The drawing under review shows one solid part. Ordinate dimensions are in mm from its lowest x, y, z. A direction names the side the tool comes from. Give positions to 0.01 mm unless a question says otherwise; leave off trailing zeros. Loops run counter-clockwise (first coordinate to the right, second up) from the corner with the lowest first, then second, coordinate; pieces in that order, holes last. Notation, with made-up numbers: M -29,81 L -11,81 A37 cw -11,117 Z; hole C -17,-24 d11. An arc over 180 degrees is marked long. One line per item, written item: value. Start each with the question number.
Q1. We need section C-C on x = 5. Write out the cut boundary in (y, z), plus the area to 3 significant figures.
Q2. We need section D-D on y = 4.5. Write out the cut boundary in (x, z), plus the area to 3 significant figures.
Q3. We need section A-A on z = 15. Write out the cut boundary in (x, y).
Q4. For pin 1 (1 mm diameter, centred on x = 15, z = 5, fed in from -Y); pin 2 (2.5 mm diameter, centred on x = 5, z = 15, fed in from +Y); pin 3 (3 mm diameter, centred on y = 15.5, z = 3.5, fed in from -X); pin 4 (2 mm diameter, centred on y = 5, z = 10.5, fed in from -X), all flat-tipped, find the tip position at first contact; note any pin that passes through.
Q5. To check wall thickness, follow line 1 along Z through (x, y) = (15, 16.75); line 2 along Z through (x, y) = (15.5, 12.5); line 3 along Y through (x, z) = (10.5, 18.25). State the ranges of each line that lie inside material, in increasing order. Write a range as from..to.
Q6. Mouldability with a two-part tool opening along X and no side actions: class the marked faces 5, 6 and 7 as released by +X, released by -X, zero draft, split by the parting line, or undercut.
Q7. We need section B-B on y = 18.75. Write out the cut boundary in (x, z).
Q8. For the marked faces 1, 2, 3 and 4, list the 3-axis set-ups (+Z, -Z, +X, -X, +Y, -Y) from which the entire face can be reached by the end or side of a thin tool; tool diameter is ignored.
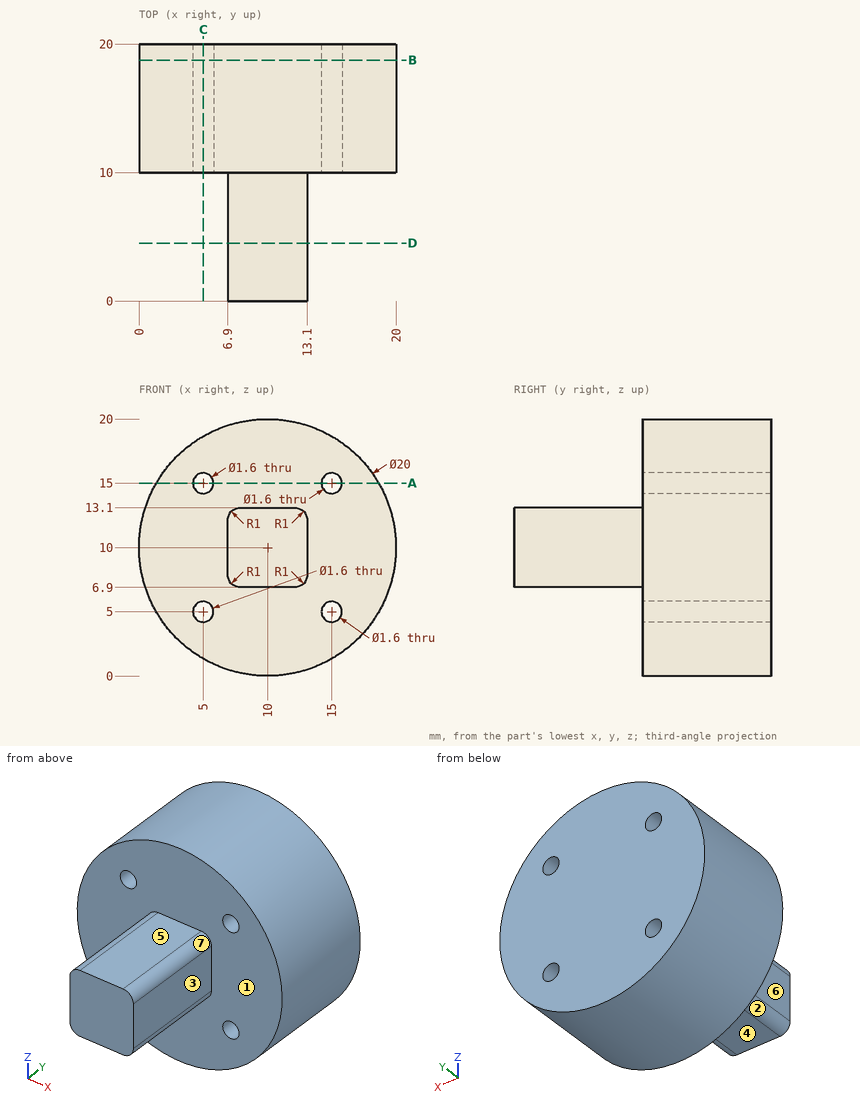
Solved:
1. outline: M 10,1.34 L 20,1.34 L 20,4.2 L 10,4.2 Z; M 10,5.8 L 20,5.8 L 20,14.2 L 10,14.2 Z; M 10,15.8 L 20,15.8 L 20,18.66 L 10,18.66 Z
1. area: 141 mm2
2. outline: M 6.9,7.9 A1 ccw 7.9,6.9 L 12.1,6.9 A1 ccw 13.1,7.9 L 13.1,12.1 A1 ccw 12.1,13.1 L 7.9,13.1 A1 ccw 6.9,12.1 Z
2. area: 37.6 mm2
3. outline: M 1.34,10 L 4.2,10 L 4.2,20 L 1.34,20 Z; M 5.8,10 L 14.2,10 L 14.2,20 L 5.8,20 Z; M 15.8,10 L 18.66,10 L 18.66,20 L 15.8,20 Z
4. pin 1: through
4. pin 2: y = 20
4. pin 3: x = 1.34
4. pin 4: x = 6.9
5. line 1: 1.34..4.2, 5.8..14.2, 15.8..18.66
5. line 2: 1.65..4.38, 5.62..14.38, 15.62..18.35
5. line 3: 10..20
6. face 5: zero draft
6. face 6: released by -X
6. face 7: released by +X
7. outline: C 10,10 d20; hole C 5,5 d1.6; hole C 5,15 d1.6; hole C 15,5 d1.6; hole C 15,15 d1.6
8. face 1: -Y
8. face 2: -Z, -X, -Y
8. face 3: +Z, -Z, +X, -Y
8. face 4: -Z, +X, -X, -Y
